Check sheet for the modelled part. Datum: model origin and axes. Units: mm. A direction names the side the tool comes from. Give positions to 0.01 mm unless a question says otherwise; leave off trailing zeros. Order: outer loops, then holes, each group sorted by start corner. A loop starts at its lowest first (then second) coordinate and runs counter-clockwise, first axis right, second up. Notation, with made-up numbers: M 79.5,32 L 85.5,32 A29 cw 85.5,67 Z; hole C -1.75,33 d4. An arc over 180 degrees is marked long. Answer in a Markdown table with one row per item. Add a question column.
from build123d import *

# Parameters (mm, degrees)
SKETCH1_W           = 61
SKETCH1_H           = 6.1
BOSS_EXTRUDE1_DEPTH = 22.5
SKETCH2_OUTSIDE_W   = 76.06
SKETCH2_OUTSIDE_H   = 21.16
SKETCH2_OUTSIDE_W_2 = 61
SKETCH2_OUTSIDE_H_2 = 5.1952
CUT_EXTRUDE1_DEPTH  = 6
CUT_EXTRUDE3_DEPTH  = 23.5
CUT_EXTRUDE4_DEPTH  = 7.1
SKETCH7_R           = 1.5
CUT_EXTRUDE5_DEPTH  = 7.1
SKETCH8_W           = 2
SKETCH8_H           = 0.06858
SKETCH8_W_2         = 6
CUT_EXTRUDE6_DEPTH  = 62


with BuildPart() as part:
    # Sketch1 → Boss-Extrude1 (new body)
    with BuildSketch(Plane(origin=(0, 0, 0), x_dir=(0, 0, -1), z_dir=(1, 0, 0))):
        with Locations((30.5, 0)):
            Rectangle(SKETCH1_W, SKETCH1_H)
    extrude(amount=BOSS_EXTRUDE1_DEPTH)

    # Sketch2 outside → Cut-Extrude1 (cut)
    with BuildSketch(Plane(origin=(22.5, 0, 0), x_dir=(0, 0, -1), z_dir=(1, 0, 0))):
        with Locations((30.5, 0)):
            Rectangle(SKETCH2_OUTSIDE_W, SKETCH2_OUTSIDE_H)
        with Locations((30.5, 0)):
            Rectangle(SKETCH2_OUTSIDE_W_2, SKETCH2_OUTSIDE_H_2, mode=Mode.SUBTRACT)
    extrude(amount=-CUT_EXTRUDE1_DEPTH, mode=Mode.SUBTRACT)

    # Sketch5 → Cut-Extrude3 (cut, through all)
    with BuildSketch(Plane.ZY):
        with BuildLine():
            Line((-43.5866, -0.1278), (-43.5866, -3.05))
            Line((-43.5866, -3.05), (-48.6514, -3.05))
            Line((-48.6514, -3.05), (-48.6514, -0.1278))
            ThreePointArc((-48.6514, -0.1278), (-46.119, 2.4046), (-43.5866, -0.1278))
        make_face()
    extrude(amount=-CUT_EXTRUDE3_DEPTH, mode=Mode.SUBTRACT)

    # Sketch6 → Cut-Extrude4 (cut, through all)
    with BuildSketch(Plane(origin=(0, 3.05, 0), x_dir=(1, 0, 0), z_dir=(0, 1, 0))):
        with BuildLine():
            Line((6, 32.9892), (9, 32.9892))
            ThreePointArc((9, 32.9892), (11.4892, 30.5), (9, 28.0108))
            Line((9, 28.0108), (6, 28.0108))
            ThreePointArc((6, 28.0108), (3.5108, 30.5), (6, 32.9892))
        make_face()
    extrude(amount=-CUT_EXTRUDE4_DEPTH, mode=Mode.SUBTRACT)

    # Sketch7 → Cut-Extrude5 (cut, through all)
    with BuildSketch(Plane(origin=(0, 3.05, 0), x_dir=(1, 0, 0), z_dir=(0, 1, 0))):
        with Locations(Location((5, 55.5, 0), (0, 0, 270))):  # turned: the seam where the file's is
            Circle(SKETCH7_R)
        with Locations(Location((5, 5.5, 0), (0, 0, 270))):  # turned: the seam where the file's is
            Circle(SKETCH7_R)
    extrude(amount=-CUT_EXTRUDE5_DEPTH, mode=Mode.SUBTRACT)

    # Sketch8 → Cut-Extrude6 (cut, through all)
    with BuildSketch(Plane.XY):
        with Locations((15.5, -3.01571)):
            Rectangle(SKETCH8_W, SKETCH8_H)
        with Locations((19.5, -2.56331)):
            Rectangle(SKETCH8_W_2, SKETCH8_H)
        with Locations((19.5, 2.56331)):
            Rectangle(SKETCH8_W_2, SKETCH8_H)
        with Locations((15.5, 3.01571)):
            Rectangle(SKETCH8_W, SKETCH8_H)
    extrude(amount=-CUT_EXTRUDE6_DEPTH, mode=Mode.SUBTRACT)


solid = part.part
Q1. Tool access check on faces 4 (the flat face through (15, 2.981, -30)), 5 (the cylindrical face through (3.51, 0.04, -30.45)), 6 (the flat face through (11, -2, -43.587)), 7 (the flat face through (11, 0, 0)), 8 (the flat face through (15, -2.981, -21)). Record the directions out of +Z, -Z, +X, -X, +Y, -Y that give a thin tool (end or side, any length) a straight path to the whole face; none if there is none.
Q2. Draft check along X on faces 1 (the flat face through (19, 2.529, -30)), 2 (the cylindrical face through (5, 0, -54)), 3 (the flat face through (0, 0, -30)). Enter one of: pulls with the +X half, pulls with the -X half, needs draft (parallel to the pull), parting line crosses it, or undercut.
Q3. Cross-section at C-C (x = 12.25). Record the boundary of the cut face in (y, z), and give its area (3 significant figures).
Q4. Thickness scan on probe 1 along Z at (x, y) = (7, -2); probe 2 along Z at (x, y) = (15.25, -0.75). Record the ranges inside material, lowest first.
Q5. Cross-section at B-B (y = -1.5). Record the boundary of the cut face in (x, z).
Q6. Go/stop test with flat-tipped pins: pin 1 (0.6 mm diameter, centred on x = 15, z = -17.5, fed in from -Y); pin 2 (1 mm diameter, centred on x = 13.5, y = -1.5, fed in from +Z); pin 3 (1 mm diameter, centred on x = 18, z = -14, fed in from +Y); pin 4 (3 mm diameter, centred on x = 19.5, z = -54, fed in from -Y). Record where each tip stops, or that it passes through.
Q7. Cross-section at D-D (z = -39). Record the boundary of the cut face in (x, y).
Q8. Cross-section at A-A (z = -30.5). Record the boundary of the cut face in (x, y), and give its area (3 significant figures).
Values follow:
| question | item | result |
|---|---|---|
| 1 | face 4 | +Z, -Z, +X, +Y |
| 1 | face 5 | +Y, -Y |
| 1 | face 6 | +X, -X, -Y |
| 1 | face 7 | +Z, +X, -X, +Y, -Y |
| 1 | face 8 | +Z, -Z, +X, -Y |
| 2 | face 1 | needs draft |
| 2 | face 2 | undercut |
| 2 | face 3 | pulls with the -X half |
| 3 | outline | M -3.05,-61 L 3.05,-61 L 3.05,0 L -3.05,0 L -3.05,-43.59 L -0.13,-43.59 A2.53 cw -0.13,-48.65 L -3.05,-48.65 Z |
| 3 | area | 347 mm² |
| 4 | probe 1 | -61 to -48.65, -43.59 to -32.99, -28.01 to 0 |
| 4 | probe 2 | -61 to -48.65, -43.59 to 0 |
| 5 | outline | M 0,-61 L 22.5,-61 L 22.5,-48.65 L 0,-48.65 Z; M 0,-43.59 L 22.5,-43.59 L 22.5,0 L 0,0 Z; hole C 5,-55.5 d3; hole C 5,-5.5 d3; hole M 6,-32.99 L 9,-32.99 A2.49 ccw 9,-28.01 L 6,-28.01 A2.49 ccw Z |
| 6 | pin 1 | y = -2.98 |
| 6 | pin 2 | z = 0 |
| 6 | pin 3 | y = 2.53 |
| 6 | pin 4 | y = -2.53 |
| 7 | outline | M 0,-3.05 L 14.5,-3.05 L 14.5,-2.98 L 16.5,-2.98 L 16.5,-2.53 L 22.5,-2.53 L 22.5,2.53 L 16.5,2.53 L 16.5,2.98 L 14.5,2.98 L 14.5,3.05 L 0,3.05 Z |
| 8 | outline | M 0,-3.05 L 3.51,-3.05 L 3.51,3.05 L 0,3.05 Z; M 11.49,-3.05 L 14.5,-3.05 L 14.5,-2.98 L 16.5,-2.98 L 16.5,-2.53 L 22.5,-2.53 L 22.5,2.53 L 16.5,2.53 L 16.5,2.98 L 14.5,2.98 L 14.5,3.05 L 11.49,3.05 Z |
| 8 | area | 82.1 mm² |
